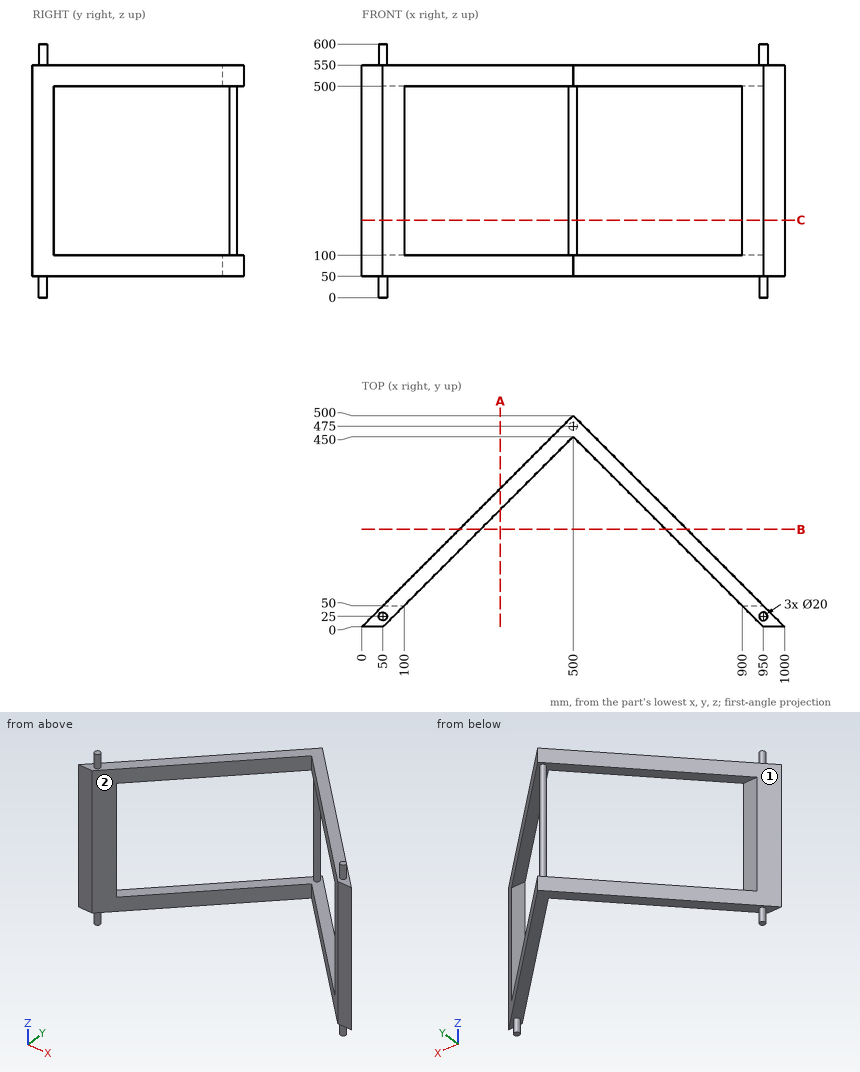
Drawing for the job (mm, zero at the part's lowest x, y, z). A direction names the side the tool comes from. Give positions to 0.01 mm unless a question says otherwise; leave off trailing zeros. Write each loop counter-clockwise with the first axis right and the second up, starting at its lowest first coordinate (ties: lowest second). Pieces come first, ordered by that corner, then holes. Notation, with made-up numbers: M -30.75,57 L 5.25,57 A16 cw 5.25,86 Z; hole C 78,89.5 d3. An arc over 180 degrees is marked long. Return JSON: item names as keys, results as strings. Group by question number.
(1) Drill centre lines: L1, parallel to Z at x = 772.5, y = 217; L2, parallel to X at y = 51, z = 519.5; L3, parallel to X at y = 337, z = 64. Where is each one in solid material? Low to high. Write a range as [from, to].
(2) Flat gauge pin, fed straight in: pin 1 Ø25 at (x, z) = (921, 310) entering from +Y. Where does the tip first touch, or does it go through?
(3) Band-saw the part on C-C (z = 183). Give the cut face in (x, y).
(4) Band-saw the part on A-A (x = 327.5). Give the cut face in (y, z), and give its area (3 significant figures).
(5) 3-axis set-ups, long thin cutter, end or side, ignore diameter. For the marked faces 1 and 2: which of +Z, -Z, +X, -X, +Y, -Y reach the whole face in a straight line?
(6) Band-saw the part on B-B (y = 231). Give the cut face in (x, z).
Entries:
{
 "1": {"L1": "z = [50, 100], [500, 550]", "L2": "x = [51, 101], [899, 949]", "L3": "x = [337, 387], [613, 663]"},
 "2": {"pin 1": "stops at y = 50"},
 "3": {"outline": "M 0,0 L 50,0 L 100,50 L 50,50 Z; C 500,475 d20; M 900,50 L 950,0 L 1000,0 L 950,50 Z"},
 "4": {"outline": "M 277.5,50 L 327.5,50 L 327.5,100 L 277.5,100 Z; M 277.5,500 L 327.5,500 L 327.5,550 L 277.5,550 Z", "area": "5,000 mm^2"},
 "5": {"face 1": "+Z, -Z, -X, +Y", "face 2": "+Z, -Z, -Y"},
 "6": {"outline": "M 231,50 L 281,50 L 281,100 L 231,100 Z; M 231,500 L 281,500 L 281,550 L 231,550 Z; M 719,50 L 769,50 L 769,100 L 719,100 Z; M 719,500 L 769,500 L 769,550 L 719,550 Z"}
}
